Could you check a few things on this model? Use its own coordinates, in mm. Give positions to 0.01 mm unless a question says otherwise; leave off trailing zeros. Loops run counter-clockwise (first coordinate to the right, second up) from the corner with the lowest first, then second, coordinate; pieces in that order, holes last. Notation, with made-up numbers: (68.25, 39.25) - (95.25, 39.25) arc R25 cw to (95.25, 74.25) - close; hole circle Ø3 at (40.25, 29). An arc over 180 degrees is marked (long way). Answer in a Markdown table with one row per item. Add a question column.
```python
from build123d import *

# Parameters (mm, degrees)
SKETCH_2_R               = 13
EXTRUDE_1_DEPTH          = 3
CUT_EXTRUDE_2_DEPTH      = 110.084751045
PATTERN_CURVE_1_DEPTH    = 3
CUT_EXTRUDE_4_DEPTH      = 110.084751045
PATTERN_CIRCULAR_1_COUNT = 6
EXTRUDE_2_DEPTH          = 3
HOLE_WIZARD_M4_1_D       = 4.2
FILLET_1_R               = 4


# Read off the part's stored shape, not the designer's step: 곡선 패턴1
with BuildPart() as part:
    # 스케치2 → 보스-돌출1 (new body)
    with BuildSketch(Plane(origin=(0, 0, 0), x_dir=(1, 0, 0), z_dir=(0, 1, 0))):
        with BuildLine():
            ThreePointArc((77.639466647, 24.999926714), (45.838842968, 27.466341176), (14.834721753, 34.956824097))
            ThreePointArc((14.834721753, 34.956824097), (0.14257607, 36.40176879), (-13.777014503, 31.48323159))
            Line((-13.777014503, 31.48323159), (-22.257495465, 26.184038948))
            ThreePointArc((-22.257495465, 26.184038948), (-35.278632699, -16.528292532), (5.235906124, -35.302354942))
            ThreePointArc((5.235906124, -35.302354942), (41.103608721, -27.588473828), (77.7, -25))
            ThreePointArc((77.7, -25), (102.699981679, 0.030266699), (77.639466647, 24.999926714))
        make_face()
        with BuildLine():
            Line((-9.539433123, 5.83088464), (-1.058952162, 11.130077283))
            ThreePointArc((-1.058952162, 11.130077283), (12.720721442, 7.948788963), (9.539433123, -5.83088464))
            Line((9.539433123, -5.83088464), (1.058952162, -11.130077283))
            ThreePointArc((1.058952162, -11.130077283), (-12.720721442, -7.948788963), (-9.539433123, 5.83088464))
        make_face(mode=Mode.SUBTRACT)
        with Locations(Location((77.7, 0, 0), (0, 0, 270))):
            Circle(SKETCH_2_R, mode=Mode.SUBTRACT)
    extrude(amount=EXTRUDE_1_DEPTH)

    # 스케치4 → 컷-돌출2 (cut, through all)
    with BuildSketch(Plane(origin=(0, 0, 0), x_dir=(-1, 0, 0), z_dir=(0, -1, 0))):
        with BuildLine():
            Line((1.82151317, -17.005644102), (10.301994131, -22.304836745))
            ThreePointArc((10.301994131, -22.304836745), (10.970064678, -25.198568201), (8.076333221, -25.866638748))
            Line((8.076333221, -25.866638748), (-0.40414774, -20.567446106))
            ThreePointArc((-0.40414774, -20.567446106), (-1.072218287, -17.673714649), (1.82151317, -17.005644102))
        make_face()
    extrude(amount=-CUT_EXTRUDE_2_DEPTH, mode=Mode.SUBTRACT)

    # 곡선 패턴1 outline → 곡선 패턴1 (cut)
    with BuildSketch(Plane(origin=(0, 0, 0), x_dir=(1, 0, 0), z_dir=(0, 1, 0))):
        with BuildLine():
            Line((24.563551451, -0.518425872), (16.08307049, -5.817618515))
            ThreePointArc((16.08307049, -5.817618515), (15.414999943, -8.711349971), (18.308731399, -9.379420519))
            Line((18.308731399, -9.379420519), (26.789212361, -4.080227876))
            ThreePointArc((26.789212361, -4.080227876), (27.457282908, -1.186496419), (24.563551451, -0.518425872))
        make_face()
        with BuildLine():
            ThreePointArc((-16.08307049, 5.817618515), (-15.414999943, 8.711349971), (-18.308731399, 9.379420519))
            Line((-18.308731399, 9.379420519), (-26.789212361, 4.080227876))
            ThreePointArc((-26.789212361, 4.080227876), (-27.457282908, 1.186496419), (-24.563551451, 0.518425872))
            Line((-24.563551451, 0.518425872), (-16.08307049, 5.817618515))
        make_face()
        with BuildLine():
            Line((8.076333221, 25.866638748), (-0.40414774, 20.567446106))
            ThreePointArc((-0.40414774, 20.567446106), (-1.072218287, 17.673714649), (1.82151317, 17.005644102))
            Line((1.82151317, 17.005644102), (10.301994131, 22.304836745))
            ThreePointArc((10.301994131, 22.304836745), (10.970064678, 25.198568202), (8.076333221, 25.866638748))
        make_face()
    extrude(amount=PATTERN_CURVE_1_DEPTH, mode=Mode.SUBTRACT)

    # 스케치5 → 컷-돌출4 (cut, through all)
    with BuildSketch(Plane(origin=(0, 0, 0), x_dir=(-1, 0, 0), z_dir=(0, -1, 0))):
        with BuildLine():
            ThreePointArc((-73.066008281, -20.072023335), (-68.831471406, -18.593256858), (-65.017373608, -16.233021524))
            ThreePointArc((-65.017373608, -16.233021524), (-64.483090846, -11.881637615), (-68.834474755, -11.347354852))
            ThreePointArc((-68.834474755, -11.347354852), (-71.500640206, -12.997228095), (-74.460704817, -14.030928933))
            ThreePointArc((-74.460704817, -14.030928933), (-76.78390375, -17.748824402), (-73.066008281, -20.072023335))
        make_face()
    cut_extrude_4 = extrude(amount=-CUT_EXTRUDE_4_DEPTH, mode=Mode.SUBTRACT)

    # 원형 패턴1: 컷-돌출4 ×6 about axis, 2 skipped
    pattern_circular_1_axis = Axis((77.7, 3, 0), (0, -1, 0))
    add([cut_extrude_4.rotate(pattern_circular_1_axis, i * 360 / PATTERN_CIRCULAR_1_COUNT) for i in range(1, PATTERN_CIRCULAR_1_COUNT) if i not in (1, 4)], mode=Mode.SUBTRACT)

    # 스케치7 → 보스-돌출2 (add)
    with BuildSketch(Plane.XZ):
        with BuildLine():
            ThreePointArc((-34.857379721, -22.180465117), (-34.155886305, -26.830127811), (-29.517020915, -27.599792717))
            Line((-29.517020915, -27.599792717), (-24.147285754, -24.913232788))
            ThreePointArc((-24.147285754, -24.913232788), (-28.457668053, -21.214942262), (-32.092293027, -16.850741341))
            Line((-32.092293027, -16.850741341), (-34.857379721, -22.180465117))
        make_face()
        with BuildLine():
            ThreePointArc((-29.517020915, 32.898985359), (-34.155886305, 32.129320453), (-34.857379721, 27.479657759))
            Line((-34.857379721, 27.479657759), (-32.092293027, 22.149933984))
            ThreePointArc((-32.092293027, 22.149933984), (-28.457668053, 26.514134904), (-24.147285754, 30.21242543))
            Line((-24.147285754, 30.21242543), (-29.517020915, 32.898985359))
        make_face()
    extrude(amount=-EXTRUDE_2_DEPTH)

    # M4 나선 코일용 탭 드릴1 (through all)
    with Locations(Plane(origin=(0, 3, 0), x_dir=(1, 0, 0), z_dir=(0, 1, 0))):
        with Locations((-31.306777179, 24.022535036), (-31.306777179, -29.321727679)):
            Hole(HOLE_WIZARD_M4_1_D / 2)

    # 필렛1
    fillet_1_edges = [part.edges().sort_by_distance(p)[0] for p in [
        (-24.147285754, 1.5, -24.913232788),
        (-32.092293027, 1.5, -16.850741341),
        (-32.092293027, 1.5, 22.149933984),
        (-24.147285754, 1.5, 30.21242543),
    ]]
    fillet(fillet_1_edges, radius=FILLET_1_R)


solid = part.part
```
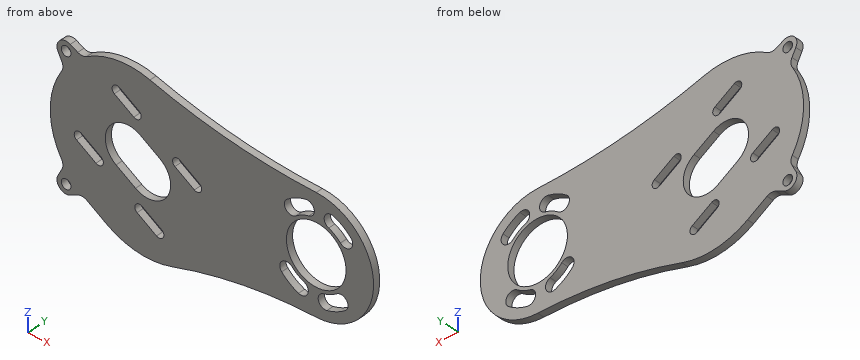
(1) I want a section at C-C on x = 59.5. Please give me the cut outline in (y, z), then the cut area to 3 significant figures.
(2) I want a section at B-B on y = 2.2. State how many separate pieces and enclosed holes the cut face has, then the cut area to 3 significant figures.
(3) Please list where these lines run through material, in increasing order: line 1 (Z direction, x = 85, y = 2.5); line 2 (X direction, y = 0.65, z = 3); line 3 (Z direction, x = 74.5, y = 1.35).
(4) I want a section at A-A on x = 37.5. Please give me the cut outline in (y, z), then the cut area to 3 significant figures.
(5) For pin 1 Ø1 at (x, y) = (5, 2) entering from +Z, with a flat end and sliding along its axis, tell me the tip position at first contact or that it passes through.
Reported:
| question | item | result |
|---|---|---|
| 1 | outline | (0, -25.78) - (3, -25.78) - (3, 25.64) - (0, 25.64) - close |
| 1 | area | 154 mm² |
| 2 | separate pieces | 1 |
| 2 | enclosed holes | 12 |
| 2 | area | 6,230 mm² |
| 3 | line 1 | -23.91 to -19.26, -12.41 to -10.76, 10.76 to 12.41, 19.24 to 23.91 |
| 3 | line 2 | -38.24 to -14.23, 12.49 to 20.59, 27.66 to 65.05, 90.35 to 102.52 |
| 3 | line 3 | -25.02 to -12.6, 12.6 to 14.04, 20.06 to 25.02 |
| 4 | outline | (0, -28.97) - (3, -28.97) - (3, 28.13) - (0, 28.13) - close |
| 4 | area | 171 mm² |
| 5 | pin 1 | z = 35.51 |
